Verification items for the finished model (mm, model axes). Face numbers are marked on the shaded views. A direction names the side the tool comes from. Coordinates: 2 decimals unless noted, no trailing zeros. Write each loop counter-clockwise with the first axis right and the second up, starting at its lowest first coordinate (ties: lowest second). Pieces come first, ordered by that corner, then holes. Notation, with made-up numbers: (78.25, 30.25) -> (84.25, 30.25) arc R20 cw to (84.25, 46.25) -> close; hole circle Ø8 at (-15.5, 57). An arc over 180 degrees is marked (long way). Write item = value, one per line. Start each with the question number.
(1) Mould release check, pull along Z, two halves, no side actions. Record for the marked faces 1, 2 and 3: released by +Z, released by -Z, zero draft, split by the parting line, or undercut.
(2) Set-up check for the marked faces 4, 5 and 6: record each of +Z, -Z, +X, -X, +Y, -Y from which the full face is reachable in a straight line by a thin tool's end or side.
(3) Section check A-A (z = 0). Record the cut outline in (x, y), plus the area to 3 significant figures.
(4) Section check B-B (y = 0.75). Record the cut outline in (x, z), plus the area to 3 significant figures.
(5) Gauge pin test, flat ends, axial feed: pin 1 Ø3 at (x, y) = (6, -5) entering from +Z; pin 2 Ø6 at (y, z) = (0, 0) entering from +X. Record the tip position at first contact, or that the pin passes through.
(6) Material ranges on probe 1 along Y at (x, z) = (5.9, 0); probe 2 along Z at (x, y) = (3.5, 4.25); probe 3 along Y at (x, z) = (2.25, -7), recorded low to high. Write a range as [from, to].
```python
from build123d import *

# Parameters (mm, degrees)
BASPROSKE_W         = 8
BASPROSKE_H         = 7.6
TOOTHCUT_DEPTH      = 14.39850738
TEETHCUTS_COUNT     = 17
TEETHCUTS_ANGLE     = 338.823529412
BORSKE_R            = 5
BORE_DEPTH          = 50.0000508
BOSS_EXTRUDE1_START = -3
SKETCH1_R           = 5
BOSS_EXTRUDE1_DEPTH = 3


with BuildPart() as part:
    # BasProSke → Base-Revolve (revolve)
    with BuildSketch(Plane(origin=(0, 0, 0), x_dir=(1, 0, 0), z_dir=(0, 1, 0)), mode=Mode.PRIVATE) as base_revolve_sk:
        with Locations((4, 3.8)):
            Rectangle(BASPROSKE_W, BASPROSKE_H)
    revolve(base_revolve_sk.sketch.rotate(Axis((-10, 0, 0), (1, 0, 0)), 180), axis=Axis((-10, 0, 0), (1, 0, 0)))

    # TooCutSke → ToothCut (cut, through all)
    with BuildSketch(Plane(origin=(0, 0, 0), x_dir=(0, 0, -1), z_dir=(1, 0, 0))):
        with BuildLine():
            ThreePointArc((0.412875903, 5.784283403), (0, 5.799), (-0.412875903, 5.784283403))
            ThreePointArc((-0.412875903, 5.784283403), (-0.662486036, 6.729558143), (-1.230208712, 7.525510726))
            ThreePointArc((-1.230208712, 7.525510726), (0, 7.6254), (1.230208712, 7.525510726))
            ThreePointArc((1.230208712, 7.525510726), (0.662486036, 6.729558143), (0.412875903, 5.784283403))
        make_face()
    toothcut = extrude(amount=TOOTHCUT_DEPTH, mode=Mode.SUBTRACT)

    # TeethCuts: ToothCut ×17 about axis
    teethcuts_axis = Axis((-10, 0, 0), (1, 0, 0))
    for i in range(1, TEETHCUTS_COUNT):
        add(toothcut.rotate(teethcuts_axis, i * TEETHCUTS_ANGLE / (TEETHCUTS_COUNT - 1)), mode=Mode.SUBTRACT)

    # BorSke → Bore (cut, symmetric)
    with BuildSketch(Plane(origin=(0, 0, 0), x_dir=(0, 0, -1), z_dir=(1, 0, 0))):
        with Locations(Location((0, 0, 0), (0, 0, 180))):
            Circle(BORSKE_R)
    extrude(amount=BORE_DEPTH, both=True, mode=Mode.SUBTRACT)

    # Sketch1 → Boss-Extrude1 (add)
    with BuildSketch(Plane.ZY.offset(BOSS_EXTRUDE1_START)):
        Circle(SKETCH1_R)
    extrude(amount=BOSS_EXTRUDE1_DEPTH)


solid = part.part
```
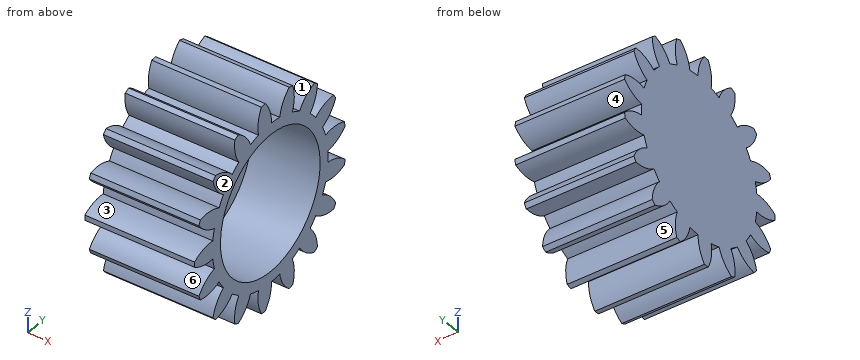
Response:
q1.face_1 = released by +Z
q1.face_2 = zero draft
q1.face_3 = undercut
q2.face_4 = +X, -X, +Y
q2.face_5 = +X, -X
q2.face_6 = +X, -X, -Y
q3.outline = (0, -7.6) -> (8, -7.6) -> (8, -5) -> (3, -5) -> (3, 5) -> (8, 5) -> (8, 5.8) -> (0, 5.8) -> close
q3.area = 57.2 mm2
q4.outline = (0, -5.75) -> (8, -5.75) -> (8, -4.94) -> (3, -4.94) -> (3, 4.94) -> (8, 4.94) -> (8, 5.75) -> (0, 5.75) -> close
q4.area = 42.6 mm2
q5.pin_1 = 6.75
q5.pin_2 = 3
q6.probe_1 = [-7.6, -5], [5, 5.8]
q6.probe_2 = [-6.11, -4.52], [-3.95, -2.63], [2.63, 3.95], [4.52, 6.11]
q6.probe_3 = [-1.12, -0.14], [1.53, 2.34]
